```python
from build123d import *

# Parameters (mm, degrees)
F0_R     = 11
F1_DEPTH = 7
F2_SIZE  = 2
F3_R     = 15
F4_R     = 3


with BuildPart() as f1:
    # F0 (on Top) → F1 (new body)
    with BuildSketch(Plane.XY):
        with BuildLine():
            ThreePointArc((11.4100490265, 9.7370827876), (12.9903810568, 7.5), (14.1375855661, 5.0128509216))
            Line((14.1375855661, 5.0128509216), (15, 4.514935716))
            Line((15, 4.514935716), (15, 8.6602540378))
            Line((15, 8.6602540378), (11.4100490265, 10.7329131988))
            Line((11.4100490265, 10.7329131988), (11.4100490265, 9.7370827876))
        make_face()
        with BuildLine():
            Line((15, 8.6602540378), (15, 4.514935716))
            Line((15, 4.514935716), (24.9852763815, -1.2500662908))
            ThreePointArc((24.9852763815, -1.2500662908), (30.2560605014, -1.2171757859), (35.2128129211, -3.0096189432))
            Line((35.2128129211, -3.0096189432), (15, 8.6602540378))
        make_face()
        with BuildLine():
            Line((-15, 4.514935716), (-14.1375855661, 5.0128509216))
            ThreePointArc((-14.1375855661, 5.0128509216), (-12.9903810568, 7.5), (-11.4100490265, 9.7370827876))
            Line((-11.4100490265, 9.7370827876), (-11.4100490265, 10.7329131988))
            Line((-11.4100490265, 10.7329131988), (-15, 8.6602540378))
            Line((-15, 8.6602540378), (-15, 4.514935716))
        make_face()
        with BuildLine():
            Line((-24.9852763815, -1.2500662908), (-15, 4.514935716))
            Line((-15, 4.514935716), (-15, 8.6602540378))
            Line((-15, 8.6602540378), (-35.2128129211, -3.0096189432))
            ThreePointArc((-35.2128129211, -3.0096189432), (-30.2560605014, -1.2171757859), (-24.9852763815, -1.2500662908))
        make_face()
        with BuildLine():
            Line((3.5899509735, -15.2478489148), (2.7275365396, -14.7499337092))
            ThreePointArc((2.7275365396, -14.7499337092), (0, -15), (-2.7275365396, -14.7499337092))
            Line((-2.7275365396, -14.7499337092), (-3.5899509735, -15.2478489148))
            Line((-3.5899509735, -15.2478489148), (0, -17.3205080757))
            Line((0, -17.3205080757), (3.5899509735, -15.2478489148))
        make_face()
        with BuildLine():
            Line((13.575227355, -21.0128509216), (3.5899509735, -15.2478489148))
            Line((3.5899509735, -15.2478489148), (0, -17.3205080757))
            Line((0, -17.3205080757), (20.2128129211, -28.9903810568))
            ThreePointArc((20.2128129211, -28.9903810568), (16.1821354021, -25.5939291197), (13.575227355, -21.0128509216))
        make_face()
        with BuildLine():
            Line((11.4100490265, 10.7329131988), (15, 8.6602540378))
            Line((15, 8.6602540378), (15, 32))
            ThreePointArc((15, 32), (14.0739250992, 26.8111049056), (11.4100490265, 22.2629172124))
            Line((11.4100490265, 22.2629172124), (11.4100490265, 10.7329131988))
        make_face()
        with BuildLine():
            ThreePointArc((35.2128129211, -3.0096189432), (30.2560605014, -1.2171757859), (24.9852763815, -1.2500662908))
            ThreePointArc((24.9852763815, -1.2500662908), (14.7224318643, -8.5), (13.575227355, -21.0128509216))
            ThreePointArc((13.575227355, -21.0128509216), (16.1821354021, -25.5939291197), (20.2128129211, -28.9903810568))
            ThreePointArc((20.2128129211, -28.9903810568), (35.2128129211, -28.9903810568), (42.7128129211, -16))
            ThreePointArc((42.7128129211, -16), (40.7031939779, -8.5), (35.2128129211, -3.0096189432))
        make_face()
        with Locations((27.7128129211, -16)):
            Circle(F0_R, mode=Mode.SUBTRACT)
        with BuildLine():
            Line((0, -17.3205080757), (-3.5899509735, -15.2478489148))
            Line((-3.5899509735, -15.2478489148), (-13.575227355, -21.0128509216))
            ThreePointArc((-13.575227355, -21.0128509216), (-16.1821354021, -25.5939291197), (-20.2128129211, -28.9903810568))
            Line((-20.2128129211, -28.9903810568), (0, -17.3205080757))
        make_face()
        with BuildLine():
            Line((-15, 32), (-15, 8.6602540378))
            Line((-15, 8.6602540378), (-11.4100490265, 10.7329131988))
            Line((-11.4100490265, 10.7329131988), (-11.4100490265, 22.2629172124))
            ThreePointArc((-11.4100490265, 22.2629172124), (-14.0739250992, 26.8111049056), (-15, 32))
        make_face()
        with BuildLine():
            ThreePointArc((-12.7128129211, -16), (-16.1821354021, -6.4060708803), (-24.9852763815, -1.2500662908))
            ThreePointArc((-24.9852763815, -1.2500662908), (-30.2560605014, -1.2171757859), (-35.2128129211, -3.0096189432))
            ThreePointArc((-35.2128129211, -3.0096189432), (-40.7031939779, -23.5), (-20.2128129211, -28.9903810568))
            ThreePointArc((-20.2128129211, -28.9903810568), (-16.1821354021, -25.5939291197), (-13.575227355, -21.0128509216))
            ThreePointArc((-13.575227355, -21.0128509216), (-12.929988707, -18.5432475803), (-12.7128129211, -16))
        make_face()
        with Locations((-27.7128129211, -16)):
            Circle(F0_R, mode=Mode.SUBTRACT)
        with BuildLine():
            Line((11, 32), (15, 32))
            ThreePointArc((15, 32), (0, 47), (-15, 32))
            Line((-15, 32), (-11, 32))
            ThreePointArc((-11, 32), (0, 43), (11, 32))
        make_face()
        with BuildLine():
            ThreePointArc((11.4100490265, 22.2629172124), (14.0739250992, 26.8111049056), (15, 32))
            Line((15, 32), (11, 32))
            ThreePointArc((11, 32), (0, 21), (-11, 32))
            Line((-11, 32), (-15, 32))
            ThreePointArc((-15, 32), (-14.0739250992, 26.8111049056), (-11.4100490265, 22.2629172124))
            ThreePointArc((-11.4100490265, 22.2629172124), (0, 17), (11.4100490265, 22.2629172124))
        make_face()
        with BuildLine():
            ThreePointArc((-11, 0), (0, 11), (11, 0))
            Line((11, 0), (15, 0))
            ThreePointArc((15, 0), (14.7828242141, 2.5432475803), (14.1375855661, 5.0128509216))
            ThreePointArc((14.1375855661, 5.0128509216), (12.9903810568, 7.5), (11.4100490265, 9.7370827876))
            ThreePointArc((11.4100490265, 9.7370827876), (9.5939291197, 11.530677519), (7.5, 12.9903810568))
            ThreePointArc((7.5, 12.9903810568), (0, 15), (-7.5, 12.9903810568))
            ThreePointArc((-7.5, 12.9903810568), (-9.5939291197, 11.530677519), (-11.4100490265, 9.7370827876))
            ThreePointArc((-11.4100490265, 9.7370827876), (-12.9903810568, 7.5), (-14.1375855661, 5.0128509216))
            ThreePointArc((-14.1375855661, 5.0128509216), (-14.7828242141, 2.5432475803), (-15, 0))
            Line((-15, 0), (-11, 0))
        make_face()
        with BuildLine():
            Line((15, 0), (11, 0))
            ThreePointArc((11, 0), (0, -11), (-11, 0))
            Line((-11, 0), (-15, 0))
            ThreePointArc((-15, 0), (-12.9903810568, -7.5), (-7.5, -12.9903810568))
            ThreePointArc((-7.5, -12.9903810568), (-5.1888950944, -14.0739250992), (-2.7275365396, -14.7499337092))
            ThreePointArc((-2.7275365396, -14.7499337092), (0, -15), (2.7275365396, -14.7499337092))
            ThreePointArc((2.7275365396, -14.7499337092), (5.1888950944, -14.0739250992), (7.5, -12.9903810568))
            ThreePointArc((7.5, -12.9903810568), (12.9903810568, -7.5), (15, 0))
        make_face()
    extrude(amount=F1_DEPTH)

    # F2
    f2_edges = [f1.edges().sort_by_distance(p)[0] for p in [
        (-11, 0, 7),
        (11, 32, 7),
        (16.712813, -16, 7),
        (16.712813, -16, 0),
        (11, 32, 0),
        (-11, 0, 0),
        (-38.712813, -16, 0),
        (-38.712813, -16, 7),
    ]]
    chamfer(f2_edges, length=F2_SIZE)

    # F3
    f3_edges = [f1.edges().sort_by_distance(p)[0] for p in [
        (0, -17.320508, 3.5),
        (15, 8.660254, 3.5),
        (-15, 8.660254, 3.5),
    ]]
    fillet(f3_edges, radius=F3_R)

    # F4
    f4_edges = [f1.edges().sort_by_distance(p)[0] for p in [
        (-11.410049, 9.737083, 3.5),
        (11.410049, 9.737083, 3.5),
        (14.137586, 5.012851, 3.5),
        (-14.137586, 5.012851, 3.5),
        (2.727537, -14.749934, 3.5),
        (-2.727537, -14.749934, 3.5),
    ]]
    fillet(f4_edges, radius=F4_R)


solid = f1.part
```
Input: part model. Units: mm. Frame: model coordinates. A direction names the side the tool comes from. Coordinates: 2 decimals unless noted, no trailing zeros. Put each result on its own line as item: value.
1. Draft query along X for faces 1 (the face through (16.955, 9.916, 3.549)), 2 (the face through (0, 47, 3)), 3 (the face through (0, 17, 3)). Return one class per face: pulls with the +X half, pulls with the -X half, needs draft (parallel to the pull), parting line crosses it, or undercut.
Report:
face 1: pulls with the +X half
face 2: parting line crosses it
face 3: undercut
2. Cut plane A-A on y = -24. State how many separate pieces and enclosed holes the cut face has, then the cut area to 3 significant figures.
Report:
separate pieces: 4
enclosed holes: 0
area: 170 mm2
3. Contact query for flat-ended pins moving along their axis: pin 1 Ø2 at (y, z) = (23, 2.5) entering from -X; pin 2 Ø1 at (x, z) = (-20, 5.5) entering from +Y; pin 3 Ø4 at (x, z) = (-33, 2.5) entering from +Y; pin 4 Ø20 at (x, y) = (0, 0) entering from -Z. Output: stop coordinate, or through.
Report:
pin 1: stops at x = -15
pin 2: stops at y = 6.61
pin 3: stops at y = -0.58
pin 4: passes through
4. Line query: line 1 along Y through (x, z) = (0, 3.25); line 2 along Y through (x, z) = (19.5, 5); line 3 along X through (y, z) = (-25.5, 6). Output: solid intervals per line, ascending.
Report:
line 1: y = -19.64 to -11, 11 to 15, 17 to 21, 43 to 47
line 2: y = -28.58 to -23.32, -8.68 to -3.45, 1.92 to 6.61
line 3: x = -39.32 to -35.04, -20.38 to -14.17, 14.17 to 20.38, 35.04 to 39.32
5. Reachability of faces 4 (the face through (-13.945, -25.372, 3.451)), 5 (the face through (0, 15, 3)), 6 (the face through (15, 25, 3)) from +Z, -Z, +X, -X, +Y, -Y: full face, straight path, thin tool, end or side. Return the list, or none.
Report:
face 4: +Z, -Z, -Y
face 5: +Z, -Z
face 6: +Z, -Z, +X, +Y
